Geometry check sheet. Reference: the model listing, model coordinates, mm. A direction names the side the tool comes from. Give positions to 0.01 mm unless a question says otherwise; leave off trailing zeros. Write each loop counter-clockwise with the first axis right and the second up, starting at its lowest first coordinate (ties: lowest second). Pieces come first, ordered by that corner, then holes.
(1) Tool access check on faces 4 (the flat face through (610, 51, -60)), 5 (the flat face through (580, 51, -17)), 6 (the flat face through (595, 49, -85)), 7 (the flat face through (610, 125, -102)), 8 (the flat face through (610, 125, -17)). Record the directions out of +Z, -Z, +X, -X, +Y, -Y that give a thin tool (end or side, any length) a straight path to the whole face; none if there is none.
(2) Depth check by flat-ended pin: P1, Ø4, axis at y = 63.5, z = -43, coming from the +X side; P2, Ø9, axis at x = 593.5, y = 52, coming from the +Z side; P3, Ø10, axis at x = 683, y = 113, coming from the -Z side. Enter the tip coordinate at first touch or a pass-through.
(3) Cross-section at C-C (x = 729). Record the boundary of the cut face in (y, z), and give its area (3 significant figures).
(4) Cross-section at D-D (y = 137.5). Record the boundary of the cut face in (x, z), and give its area (3 significant figures).
(5) Mould release check, pull along X, two halves, no side actions. Record for faces 1 (the flat face through (580, 51, -102)), 2 (the flat face through (348, 150, -59)), 3 (the flat face through (833.652, 125.35, -41.338)): +X half, -X half, draft (parallel to the pull), parting line (faces both ways), or undercut.
(6) Cross-section at B-B (z = -105.5). Record the boundary of the cut face in (x, y).
(7) Thickness scan on line 1 along X through (y, z) = (67, -5.5); line 2 along X through (y, z) = (65, -62); line 3 along Z through (x, y) = (779, 106). Record the ranges inside material, lowest first.
(8) Cross-section at A-A (y = 74). Record the boundary of the cut face in (x, z), and give its area (3 significant figures).
```python
from build123d import *

# Parameters (mm, degrees)
SKETCH_1_W          = 120
SKETCH_1_H          = 150
EXTRUDE_1_DEPTH     = 610
SKETCH_2_W          = 50
SKETCH_2_H          = 50
EXTRUDE_2_DEPTH     = 300
SKETCH_3_W          = 60
SKETCH_3_H          = 90
EXTRUDE_3_DEPTH     = 140
SKETCH_4_W          = 35
SKETCH_4_H          = 100
CUT_EXTRUDE_1_DEPTH = 30
CUT_EXTRUDE_2_DEPTH = 151


with BuildPart() as part:
    # 草图1 → 凸台-拉伸1 (new body)
    with BuildSketch(Plane(origin=(0, 0, 0), x_dir=(0, 0, -1), z_dir=(1, 0, 0))):
        with Locations((60, 75)):
            Rectangle(SKETCH_1_W, SKETCH_1_H)
    extrude(amount=EXTRUDE_1_DEPTH)

    # 草图2 → 凸台-拉伸2 (add)
    with BuildSketch(Plane(origin=(610, 0, 0), x_dir=(0, 0, -1), z_dir=(1, 0, 0))):
        with Locations((60, 125)):
            Rectangle(SKETCH_2_W, SKETCH_2_H)
    extrude(amount=EXTRUDE_2_DEPTH)

    # 草图3 → 凸台-拉伸3 (add)
    with BuildSketch(Plane.ZY):
        with Locations((-60, 75)):
            Rectangle(SKETCH_3_W, SKETCH_3_H)
    extrude(amount=EXTRUDE_3_DEPTH)

    # 草图4 → 切除-拉伸1 (cut)
    with BuildSketch(Plane(origin=(610, 0, 0), x_dir=(0, 0, -1), z_dir=(1, 0, 0))):
        with Locations((17.5, 50)):
            Rectangle(SKETCH_4_W, SKETCH_4_H)
        with Locations((102.5, 50)):
            Rectangle(SKETCH_4_W, SKETCH_4_H)
    extrude(amount=-CUT_EXTRUDE_1_DEPTH, mode=Mode.SUBTRACT)

    # 草图5 → 切除-拉伸2 (cut, through all)
    with BuildSketch(Plane(origin=(0, 150, 0), x_dir=(1, 0, 0), z_dir=(0, 1, 0))):
        Polygon((810, 35), (860, 35), (856.650635095, 47.5), align=None)
        Polygon((881.650635095, 72.5), (885, 85), (835, 85), align=None)
    extrude(amount=-CUT_EXTRUDE_2_DEPTH, mode=Mode.SUBTRACT)


solid = part.part
```
Reply:
1. face 4: +Z, -Z, +X, -Y
1. face 5: +Z, +X, -Y
1. face 6: -Z, +X, -Y
1. face 7: -Z, +X, +Y, -Y
1. face 8: +Z, +X, +Y, -Y
2. P1: stops at x = 610
2. P2: stops at z = -35
2. P3: stops at z = -85
3. outline: (100, -85) - (150, -85) - (150, -35) - (100, -35) - close
3. area: 2,500 mm2
4. outline: (0, -120) - (610, -120) - (610, -85) - (835, -85) - (881.65, -72.5) - (885, -85) - (910, -85) - (910, -35) - (860, -35) - (856.65, -47.5) - (810, -35) - (610, -35) - (610, 0) - (0, 0) - close
4. area: 87,600 mm2
5. face 1: +X half
5. face 2: draft
5. face 3: undercut
6. outline: (0, 0) - (580, 0) - (580, 100) - (610, 100) - (610, 150) - (0, 150) - close
7. line 1: x = 0 to 580
7. line 2: x = -140 to 610
7. line 3: z = -85 to -35
8. outline: (-140, -90) - (0, -90) - (0, -120) - (580, -120) - (580, -85) - (610, -85) - (610, -35) - (580, -35) - (580, 0) - (0, 0) - (0, -30) - (-140, -30) - close
8. area: 79,500 mm2
